Check sheet for the modelled part. Datum: model origin and axes. Units: mm. Face numbers are marked on the shaded views. A direction names the side the tool comes from. Give positions to 0.01 mm unless a question says otherwise; leave off trailing zeros. Write each loop counter-clockwise with the first axis right and the second up, starting at its lowest first coordinate (ties: lowest second). Pieces come first, ordered by that corner, then holes. Notation, with made-up numbers: M 75.25,22.5 L 117.25,22.5 A31 ccw 117.25,60.5 Z; hole C 75,-27 d3. An arc over 180 degrees is marked long. One line per item, written item: value. Start each with the question number.
from build123d import *

# Parameters (mm, degrees)
F0_W      = 30.8750208
F0_H      = 72.8625058
F0_R      = 2.2479
F0_R_2    = 5.9124977
F1_DEPTH  = 3.437509
F2_W      = 30.8750208
F2_H      = 72.8625058
F2_R      = 2.2479
F2_R_2    = 7.5
F3_DEPTH  = 12
F4_W      = 24
F4_H      = 15
F5_DEPTH  = 7.5
F6_R      = 7.49999
F8_DEPTH  = 30.8750208
F9_R      = 3.96875
F10_DEPTH = 9.0875104
F11_R     = 3.96875
F12_R     = 1.7272
F13_DEPTH = 6.35
F14_SIZE  = 1.850009


# Not quite as in the source:
# - a fillet or chamfer is up to 0.001 mm smaller than in the source, because OpenCascade refuses the exact size


with BuildPart() as f1:
    # F0 (on Top) → F1 (new body)
    with BuildSketch(Plane.XY):
        with Locations((15.4375104, -36.4312529)):
            Rectangle(F0_W, F0_H)
        with Locations((15.4375104, -49.1312477)):
            Circle(F0_R, mode=Mode.SUBTRACT)
        with Locations((15.4375104, -23.7312477)):
            Circle(F0_R, mode=Mode.SUBTRACT)
        with Locations((15.4375104, -10.6749977)):
            Circle(F0_R_2, mode=Mode.SUBTRACT)
    extrude(amount=F1_DEPTH)

    # F2 (on face) → F3 (join)
    with BuildSketch(Plane.XY.offset(3.437509)):
        with Locations((15.4375104, -36.4312529)):
            Rectangle(F2_W, F2_H)
        with Locations((15.4375104, -49.1312477)):
            Circle(F2_R, mode=Mode.SUBTRACT)
        with Locations((15.4375104, -23.7312477)):
            Circle(F2_R, mode=Mode.SUBTRACT)
        with Locations((15.4375104, -10.6749977)):
            Circle(F2_R_2, mode=Mode.SUBTRACT)
    extrude(amount=F3_DEPTH)

    # F4 (on face) → F5 (cut)
    with BuildSketch(Plane.XY.offset(15.437509)):
        with Locations((15.4375104, -62.1875058)):
            Rectangle(F4_W, F4_H)
    extrude(amount=-F5_DEPTH, mode=Mode.SUBTRACT)

    # F6 (radius 7.5 in the source; OpenCascade refuses exactly that, so slightly less here)
    f6_edges = [f1.edges().sort_by_distance(p)[0] for p in [
        (15.43751, -54.687506, 7.937509),
        (15.43751, -69.687506, 7.937509),
    ]]
    fillet(f6_edges, radius=F6_R)

    # F7 (on face) → F8 (cut, through all)
    with BuildSketch(Plane(origin=(0, 0, 0), x_dir=(0, -1, 0), z_dir=(-1, 0, 0))):
        with BuildLine():
            Line((68.1000035, 15.437509), (56.2750081, 15.437509))
            ThreePointArc((56.2750081, 15.437509), (62.1875058, 9.5250113), (68.1000035, 15.437509))
        make_face()
    extrude(amount=-F8_DEPTH, mode=Mode.SUBTRACT)

    # F9 (on face) → F10 (cut)
    with BuildSketch(Plane(origin=(0, 0, 0), x_dir=(1, 0, 0), z_dir=(0, 0, -1))):
        with Locations((15.4375104, 23.7312477)):
            Circle(F9_R)
        with Locations((15.4375104, 49.1312477)):
            Circle(F9_R)
    extrude(amount=-F10_DEPTH, mode=Mode.SUBTRACT)

    # F11
    f11_edges = [f1.edges().sort_by_distance(p)[0] for p in [
        (0, -36.431253, 0),
        (30.875021, -36.431253, 0),
    ]]
    fillet(f11_edges, radius=F11_R)

    # F12 (on face) → F13 (cut)
    with BuildSketch(Plane.XZ.offset(72.8625058)):
        with Locations((3.96875, 3.96875)):
            Circle(F12_R)
    extrude(amount=-F13_DEPTH, mode=Mode.SUBTRACT)

    # F14
    f14_edges = [f1.edges().sort_by_distance(p)[0] for p in [
        (9.525013, -10.674998, 0),
        (30.875021, -62.187506, 9.525011),
        (0, -62.187506, 9.525011),
    ]]
    chamfer(f14_edges, length=F14_SIZE)


solid = f1.part
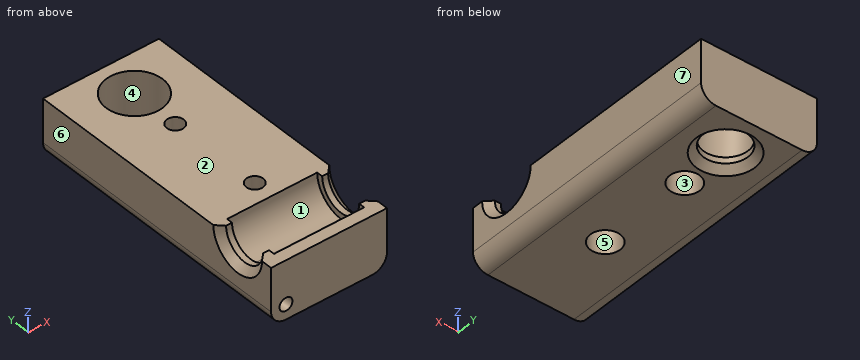
1) Cross-section at B-B (z = 6.5). Record the boundary of the cut face in (x, y) (1 decimal).
2) Gauge pin test, flat ends, axial feed: pin 1 (4 mm diameter, centred on x = 15.44, y = -49.13, fed in from +Z); pin 2 (7 mm diameter, centred on x = 15.44, y = -23.73, fed in from -Z); pin 3 (6 mm diameter, centred on y = -64, z = 12, fed in from -X); pin 4 (2.5 mm diameter, centred on y = -63, z = 10, fed in from +X). Record the tip position at first contact, or that the pin passes through.
3) Material ranges on L1, parallel to Y at x = 15.5, z = 6; L2, parallel to Y at x = 13.5, z = 6.5; L3, parallel to Y at x = 17.5, z = 10, recorded low to high. Write a range as from..to.
4) Tool access check on the marked faces 1, 2 and 3. Record the directions out of +Z, -Z, +X, -X, +Y, -Y that give a thin tool (end or side, any length) a straight path to the whole face; none if there is none.
5) Cross-section at C-C (z = 13). State how many separate pieces and enclosed holes the cut face has, plus the area to 3 significant figures.
6) Draft check along X on the marked faces 4, 5, 6 and 7. Enter one of: released by +X, released by -X, zero draft, split by the parting line, or undercut.
Data:
1. outline: M 0,-72.9 L 30.9,-72.9 L 30.9,0 L 0,0 Z; hole C 15.4,-10.7 d15; hole C 15.4,-49.1 d7.9; hole C 15.4,-23.7 d7.9
2. pin 1: passes through
2. pin 2: stops at z = 9.09
2. pin 3: stops at x = 0.88
2. pin 4: stops at x = 29.86
3. L1: y = -72.86..-53.1, -45.16..-27.7, -19.76..-18.17, -3.18..0
3. L2: y = -72.86..-52.59, -45.67..-27.19, -20.27..-17.92, -3.43..0
3. L3: y = -72.86..-67.35, -57.02..-50.03, -48.24..-24.63, -22.84..-17.89, -3.46..0
4. face 1: +Z
4. face 2: +Z, +X, -X, +Y, -Y
4. face 3: -Z
5. separate pieces: 2
5. enclosed holes: 3
5. area: 1,620 mm2
6. face 4: undercut
6. face 5: undercut
6. face 6: released by -X
6. face 7: released by +X
